from build123d import *

# Parameters (mm, degrees)
SKETCH1_W             = 12.7
SKETCH1_H             = 12.7
BOSS_EXTRUDE1_DEPTH   = 114.3
BOSS_EXTRUDE1_2_DEPTH = 114.3
SKETCH2_W             = 12.7
SKETCH2_H             = 12.7
BOSS_EXTRUDE2_DEPTH   = 228.6
SKETCH3_W             = 101.6
SKETCH3_H             = 12.7
BOSS_EXTRUDE3_DEPTH   = 114.3
SKETCH4_R             = 1.397
CUT_EXTRUDE1_DEPTH    = 12.7
BOSS_EXTRUDE4_DEPTH   = 12.7
CUT_EXTRUDE2_DEPTH    = 12.7
SKETCH7_W             = 63.5
SKETCH7_H             = 83.82
CUT_EXTRUDE3_DEPTH    = 12.7


with BuildPart() as part:
    # Sketch1 → Boss-Extrude1 (new body)
    with BuildSketch(Plane(origin=(0, 0, 0), x_dir=(1, 0, 0), z_dir=(0, 1, 0))):
        with Locations((-107.95, -6.35)):
            Rectangle(SKETCH1_W, SKETCH1_H)
    extrude(amount=BOSS_EXTRUDE1_DEPTH)



with BuildPart() as body_2:
    # Sketch1 → Boss-Extrude1 2 (new body)
    with BuildSketch(Plane(origin=(0, 0, 0), x_dir=(1, 0, 0), z_dir=(0, 1, 0))):
        with Locations((107.95, -6.35)):
            Rectangle(SKETCH1_W, SKETCH1_H)
    extrude(amount=BOSS_EXTRUDE1_2_DEPTH)


with BuildPart() as part_1:
    add(part.part)

    add(body_2.part)  # Boss-Extrude2 merges body 2
    # Sketch2 → Boss-Extrude2 (add)
    with BuildSketch(Plane.ZY.offset(114.3)):
        with Locations((6.35, 120.65)):
            Rectangle(SKETCH2_W, SKETCH2_H)
    extrude(amount=-BOSS_EXTRUDE2_DEPTH)

    # Sketch3 → Boss-Extrude3 (add)
    with BuildSketch(Plane.XZ.offset(-114.3)):
        with Locations((0, 6.35)):
            Rectangle(SKETCH3_W, SKETCH3_H)
    extrude(amount=BOSS_EXTRUDE3_DEPTH)

    # Sketch4 → Cut-Extrude1 (cut)
    with BuildSketch(Plane(origin=(114.3, 0, 0), x_dir=(0, 0, -1), z_dir=(1, 0, 0))):
        with Locations((-6.35, 4.445)):
            Circle(SKETCH4_R)
    cut_extrude1 = extrude(amount=-CUT_EXTRUDE1_DEPTH, mode=Mode.SUBTRACT)

    # Mirror1: Cut-Extrude1 across plane
    add(cut_extrude1.mirror(Plane(origin=(0, 0, 0), x_dir=(0, 0, 1), z_dir=(1, 0, 0))), mode=Mode.SUBTRACT)

    # Sketch5 → Boss-Extrude4 (add)
    with BuildSketch(Plane(origin=(0, 0, 0), x_dir=(-1, 0, 0), z_dir=(0, 0, -1))):
        with BuildLine():
            Line((-101.6, 114.3), (-101.6, 101.6))
            ThreePointArc((-101.6, 101.6), (-97.880256121, 110.580256121), (-88.9, 114.3))
            Line((-88.9, 114.3), (-101.6, 114.3))
        make_face()
        with BuildLine():
            Line((-50.8, 114.3), (-63.5, 114.3))
            ThreePointArc((-63.5, 114.3), (-54.519743879, 110.580256121), (-50.8, 101.6))
            Line((-50.8, 101.6), (-50.8, 114.3))
        make_face()
    boss_extrude4 = extrude(amount=-BOSS_EXTRUDE4_DEPTH)

    # Mirror2: Boss-Extrude4 across plane
    add(boss_extrude4.mirror(Plane(origin=(0, 0, 0), x_dir=(0, 0, 1), z_dir=(1, 0, 0))))

    # Sketch6 → Cut-Extrude2 (cut)
    with BuildSketch(Plane(origin=(0, 0, 0), x_dir=(-1, 0, 0), z_dir=(0, 0, -1))):
        with BuildLine():
            Line((-114.3, 127), (-114.3, 114.3))
            ThreePointArc((-114.3, 114.3), (-110.580256121, 123.280256121), (-101.6, 127))
            Line((-101.6, 127), (-114.3, 127))
        make_face()
    cut_extrude2 = extrude(amount=-CUT_EXTRUDE2_DEPTH, mode=Mode.SUBTRACT)

    # Mirror3: Cut-Extrude2 across plane
    add(cut_extrude2.mirror(Plane(origin=(0, 0, 0), x_dir=(0, 0, 1), z_dir=(1, 0, 0))), mode=Mode.SUBTRACT)

    # Sketch7 → Cut-Extrude3 (cut)
    with BuildSketch(Plane(origin=(0, 0, 0), x_dir=(-1, 0, 0), z_dir=(0, 0, -1))):
        with Locations((0, 66.04)):
            Rectangle(SKETCH7_W, SKETCH7_H)
    extrude(amount=-CUT_EXTRUDE3_DEPTH, mode=Mode.SUBTRACT)


solid = part_1.part
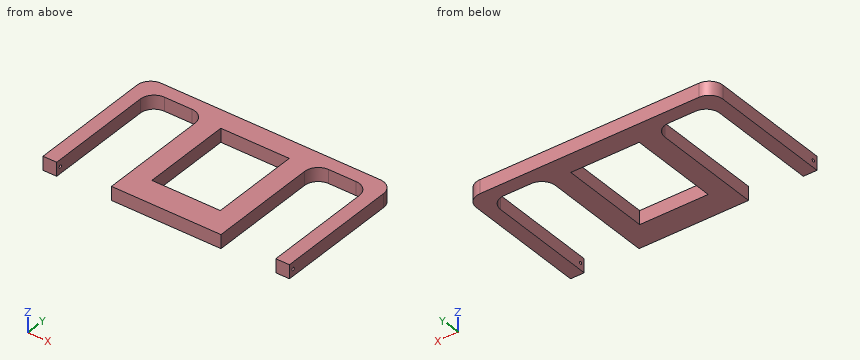
Read the model definition and answer for the solid it produces. Units are mm, in the model's axes. Round coordinates to 2 decimals unless told otherwise and drop trailing zeros. Write each loop counter-clockwise with the first axis right and the second up, starting at its lowest first coordinate (ties: lowest second). Pieces come first, ordered by that corner, then holes.
Q1. A flat-ended cylindrical pin translates along its axis: P1, Ø6.5, axis at x = -77, z = 6, coming from the -Y side. Find the tip coordinate at first contact, or state that the pin passes through.
Values:
P1: stops at y = 114.3
Q2. Straight lines are drawn through the part: line 1 (X direction, y = 62, z = 4.75); line 2 (X direction, y = 13, z = 3.25); line 3 (Y direction, x = 84.5, z = 6). For each, find the intervals that lie inside material, in ascending order.
Values:
line 1: x = -114.3 to -101.6, -50.8 to -31.75, 31.75 to 50.8, 101.6 to 114.3
line 2: x = -114.3 to -101.6, -50.8 to 50.8, 101.6 to 114.3
line 3: y = 114.3 to 127
Q3. Find section A-A on x = -28. Determine the outline of the cut face in (y, z), and give its area (3 significant figures).
Values:
outline: (0, 0) - (24.13, 0) - (24.13, 12.7) - (0, 12.7) - close; (107.95, 0) - (127, 0) - (127, 12.7) - (107.95, 12.7) - close
area: 548 mm2
Q4. Find section B-B on y = 9. Determine the outline of the cut face in (x, z).
Values:
outline: (-114.3, 0) - (-101.6, 0) - (-101.6, 12.7) - (-114.3, 12.7) - close; (-50.8, 0) - (50.8, 0) - (50.8, 12.7) - (-50.8, 12.7) - close; (101.6, 0) - (114.3, 0) - (114.3, 12.7) - (101.6, 12.7) - close
Q5. Find section D-D on x = 86. Determine the outline of the cut face in (y, z).
Values:
outline: (114.3, 0) - (127, 0) - (127, 12.7) - (114.3, 12.7) - close
Q6. Find section C-C on y = 73. Determine the outline of the cut face in (x, z).
Values:
outline: (-114.3, 0) - (-101.6, 0) - (-101.6, 12.7) - (-114.3, 12.7) - close; (-50.8, 0) - (-31.75, 0) - (-31.75, 12.7) - (-50.8, 12.7) - close; (31.75, 0) - (50.8, 0) - (50.8, 12.7) - (31.75, 12.7) - close; (101.6, 0) - (114.3, 0) - (114.3, 12.7) - (101.6, 12.7) - close
